Check sheet for the modelled part. Datum: model origin and axes. Units: mm. A direction names the side the tool comes from. Round coordinates to 2 decimals unless told otherwise and drop trailing zeros. Put each result on its own line as item: value. Start each with the question number.
```python
from build123d import *

# Parameters (mm, degrees)
SKETCH2_R           = 19.3
SKETCH2_R_2         = 17.8
BOSS_EXTRUDE1_DEPTH = 8
SKETCH2_3_R         = 20.3
SKETCH2_3_R_2       = 19.3
BOSS_EXTRUDE2_DEPTH = 1
BOSS_EXTRUDE3_START = 7
SKETCH2_4_R         = 20.3
SKETCH2_4_R_2       = 19.3
BOSS_EXTRUDE3_DEPTH = 1
BOSS_EXTRUDE4_START = -2
SKETCH3_R           = 17.8
SKETCH3_R_2         = 7.55
BOSS_EXTRUDE4_DEPTH = 2
BOSS_EXTRUDE5_START = 4
SKETCH4_R           = 11.25
SKETCH4_R_2         = 7.55
SKETCH4_R_3         = 1
BOSS_EXTRUDE5_DEPTH = 4
SKETCH5_R           = 1
CUT_EXTRUDE1_DEPTH  = 6
SKETCH6_R           = 2
CUT_EXTRUDE2_DEPTH  = 1
FILLET1_SIZE        = 2


with BuildPart() as part:
    # Sketch2 → Boss-Extrude1 (new body)
    with BuildSketch(Plane(origin=(0, 0, 0), x_dir=(1, 0, 0), z_dir=(0, 1, 0))):
        with Locations(Location((0, 0, 0), (0, 0, 270))):
            Circle(SKETCH2_R)
        with Locations(Location((0, 0, 0), (0, 0, 270))):
            Circle(SKETCH2_R_2, mode=Mode.SUBTRACT)
    extrude(amount=BOSS_EXTRUDE1_DEPTH)

    # Sketch2<3> → Boss-Extrude2 (add)
    with BuildSketch(Plane(origin=(0, 0, 0), x_dir=(1, 0, 0), z_dir=(0, 1, 0))):
        with Locations(Location((0, 0, 0), (0, 0, 270))):
            Circle(SKETCH2_3_R)
        with Locations(Location((0, 0, 0), (0, 0, 270))):
            Circle(SKETCH2_3_R_2, mode=Mode.SUBTRACT)
    extrude(amount=BOSS_EXTRUDE2_DEPTH)

    # Sketch2<4> → Boss-Extrude3 (add)
    with BuildSketch(Plane(origin=(0, 0, 0), x_dir=(1, 0, 0), z_dir=(0, 1, 0)).offset(BOSS_EXTRUDE3_START)):
        with Locations(Location((0, 0, 0), (0, 0, 270))):
            Circle(SKETCH2_4_R)
        with Locations(Location((0, 0, 0), (0, 0, 270))):
            Circle(SKETCH2_4_R_2, mode=Mode.SUBTRACT)
    extrude(amount=BOSS_EXTRUDE3_DEPTH)

    # Sketch3 → Boss-Extrude4 (add)
    with BuildSketch(Plane(origin=(0, 8, 0), x_dir=(1, 0, 0), z_dir=(0, 1, 0)).offset(BOSS_EXTRUDE4_START)):
        with Locations(Location((0, 0, 0), (0, 0, 270))):
            Circle(SKETCH3_R)
        with Locations(Location((0, 0, 0), (0, 0, 270))):
            Circle(SKETCH3_R_2, mode=Mode.SUBTRACT)
    extrude(amount=BOSS_EXTRUDE4_DEPTH)

    # Sketch4 → Boss-Extrude5 (add)
    with BuildSketch(Plane.XZ.offset(-6).offset(BOSS_EXTRUDE5_START)):
        with Locations(Location((0, 0, 0), (0, 0, 90))):
            Circle(SKETCH4_R)
        with Locations(Location((0, 0, 0), (0, 0, 90))):
            Circle(SKETCH4_R_2, mode=Mode.SUBTRACT)
        with Locations(Location((0, 9.2, 0), (0, 0, 270))):
            Circle(SKETCH4_R_3, mode=Mode.SUBTRACT)
        with Locations(Location((7.967433715, 4.6, 0), (0, 0, 270))):
            Circle(SKETCH4_R_3, mode=Mode.SUBTRACT)
        with Locations(Location((7.967433715, -4.6, 0), (0, 0, 270))):
            Circle(SKETCH4_R_3, mode=Mode.SUBTRACT)
        with Locations(Location((0, -9.2, 0), (0, 0, 270))):
            Circle(SKETCH4_R_3, mode=Mode.SUBTRACT)
        with Locations(Location((-7.967433715, -4.6, 0), (0, 0, 270))):
            Circle(SKETCH4_R_3, mode=Mode.SUBTRACT)
        with Locations(Location((-7.967433715, 4.6, 0), (0, 0, 270))):
            Circle(SKETCH4_R_3, mode=Mode.SUBTRACT)
    extrude(amount=-BOSS_EXTRUDE5_DEPTH)

    # Sketch5 → Cut-Extrude1 (cut)
    with BuildSketch(Plane.XZ.offset(-2)):
        with Locations(Location((0, 9.2, 0), (0, 0, 90))):
            Circle(SKETCH5_R)
        with Locations(Location((7.967433715, 4.6, 0), (0, 0, 90))):
            Circle(SKETCH5_R)
        with Locations(Location((7.967433715, -4.6, 0), (0, 0, 90))):
            Circle(SKETCH5_R)
        with Locations(Location((0, -9.2, 0), (0, 0, 90))):
            Circle(SKETCH5_R)
        with Locations(Location((-7.967433715, -4.6, 0), (0, 0, 90))):
            Circle(SKETCH5_R)
        with Locations(Location((-7.967433715, 4.6, 0), (0, 0, 90))):
            Circle(SKETCH5_R)
    extrude(amount=-CUT_EXTRUDE1_DEPTH, mode=Mode.SUBTRACT)

    # Sketch6 → Cut-Extrude2 (cut)
    with BuildSketch(Plane(origin=(0, 8, 0), x_dir=(1, 0, 0), z_dir=(0, 1, 0))):
        with Locations((0, -9.2)):
            Circle(SKETCH6_R)
        with Locations((-7.967433715, -4.6)):
            Circle(SKETCH6_R)
        with Locations((-7.967433715, 4.6)):
            Circle(SKETCH6_R)
        with Locations((0, 9.2)):
            Circle(SKETCH6_R)
        with Locations((7.967433715, 4.6)):
            Circle(SKETCH6_R)
        with Locations((7.967433715, -4.6)):
            Circle(SKETCH6_R)
    extrude(amount=-CUT_EXTRUDE2_DEPTH, mode=Mode.SUBTRACT)

    # Fillet1
    # a fillet whose section is not a circle: 2 mm, written as the material it adds along each edge
    with BuildSketch(Plane(origin=(0, 6, 0), x_dir=(0, 0, 1), z_dir=(-1, 0, 0))) as fillet1_piece_1:
        with BuildLine():
            Bezier((17.8, -FILLET1_SIZE), (17.8, 0), (17.8 - FILLET1_SIZE, 0), weights=[1, 0.19047619, 1])
            Line((17.8 - FILLET1_SIZE, 0), (17.8, 0))
            Line((17.8, 0), (17.8, -FILLET1_SIZE))
        make_face()
    revolve(axis=Axis((0, 6, 0), (0, 1, 0)))
    with BuildSketch(Plane(origin=(0, 6, 0), x_dir=(0, 0, 1), z_dir=(1, 0, 0))) as fillet1_piece_2:
        with BuildLine():
            Bezier((11.25 + FILLET1_SIZE, 0), (11.25, 0), (11.25, FILLET1_SIZE), weights=[1, 0.19047619, 1])
            Line((11.25, FILLET1_SIZE), (11.25, 0))
            Line((11.25, 0), (11.25 + FILLET1_SIZE, 0))
        make_face()
    revolve(axis=Axis((0, 6, 0), (0, -1, 0)))


solid = part.part
```
Q1. Draft check along X on faces 6 (the face through (-16.45, 7, 10.43)), 7 (the face through (-7.78, 0.49, 18.75)), 8 (the face through (1, 7, 10)), 9 (the face through (0.998, 4.465, 9.134)). Enter one of: +X half, -X half, draft (parallel to the pull), parting line (faces both ways), or undercut.
Q2. Material ranges on line 1 (X direction, y = 4.25, z = -9); line 2 (X direction, y = 5.35, z = -9.2); line 3 (Y direction, x = -9.5, z = 2), recorded low to high. Write a range as from..to.
Q3. Set-up check for faces 1 (the face through (-9.735, 7.507, 5.536)), 2 (the face through (8.965, 4.465, 4.534)), 3 (the face through (-9, 8, 0)), 4 (the face through (-13, 6, -4)), 5 (the face through (19.136, 3.958, -2.512)): record each of +Z, -Z, +X, -X, +Y, -Y from which the full face is reachable in a straight line by a thin tool's end or side.
Q4. Depth check by flat-ended pin: pin 1 Ø3 at (x, z) = (-7.97, 4.6) entering from -Y; pin 2 Ø1 at (y, z) = (3.5, -9) entering from -X; pin 3 Ø1.6 at (x, z) = (-7.97, 4.6) entering from +Y; pin 4 Ø3 at (y, z) = (3.5, -7) entering from -X. Enter the tip coordinate at first touch or a pass-through.
Q5. Cross-section at A-A on y = 3. State how many separate pieces and enclosed holes the cut face has, and give its area (3 significant figures).
Answer list:
1. face 6: draft
1. face 7: parting line
1. face 8: undercut
1. face 9: undercut
2. line 1: x = -17.07..-15.25, -6.91..-0.98, 0.98..6.91, 15.25..17.07
2. line 2: x = -16.97..-14.01, -8.14..-1, 1..8.14, 14.01..16.97
2. line 3: y = 2..8
3. face 1: +Y
3. face 2: +Y, -Y
3. face 3: +Z, -Z, +X, -X, +Y
3. face 4: -Y
3. face 5: none
4. pin 1: stops at y = 2
4. pin 2: stops at x = -17.33
4. pin 3: passes through
4. pin 4: stops at x = -18.5
5. separate pieces: 2
5. enclosed holes: 8
5. area: 375 mm2
